Study the drawing (mm; zero at the part's minimum x, y, z) and answer. Round coordinates to 2 decimals unless told otherwise and drop trailing zeros. Order: outer loops, then holes, each group sorted by start corner. A loop starts at its lowest first (then second) coordinate and runs counter-clockwise, first axis right, second up. Notation, with made-up numbers: (-28, 31) - (-10, 31) arc R17 ccw to (-10, 38) - close; hole circle Ø7 at (-15.5, 8). An arc over 180 degrees is marked (long way). Put each result on its own line as item: value.
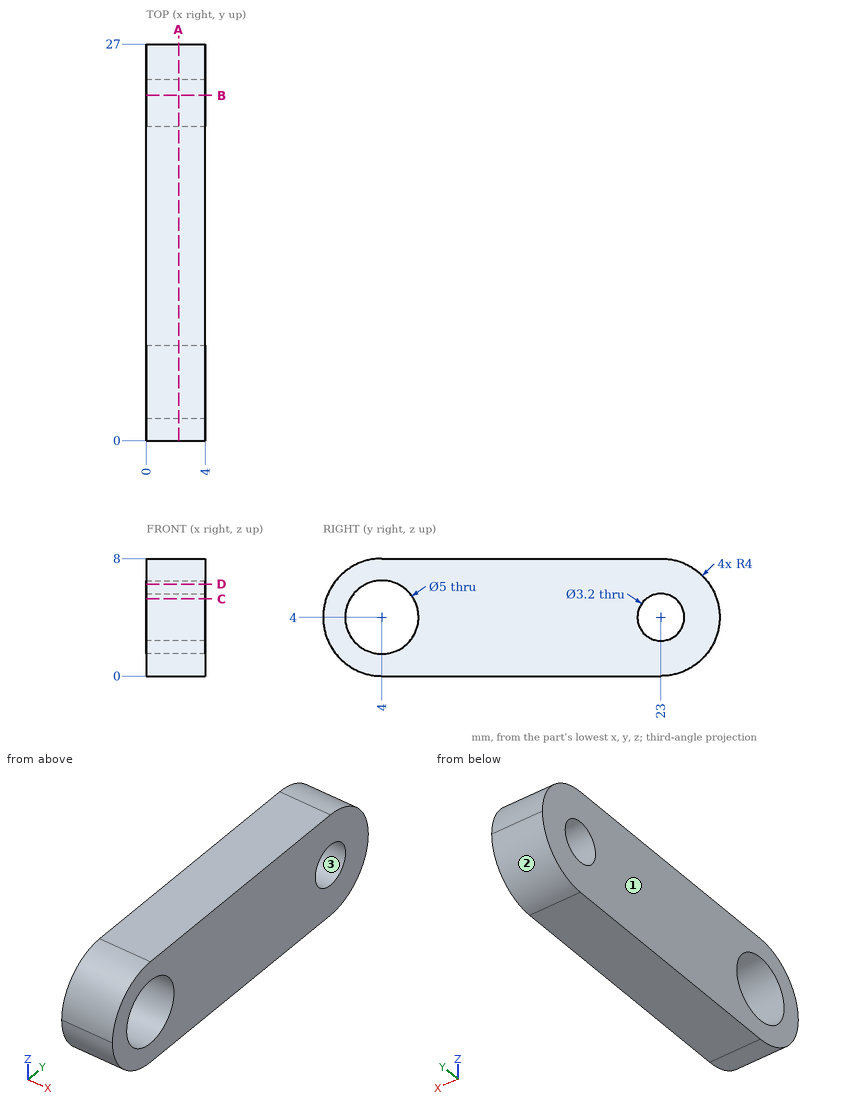
1) A cutting plane is placed at D-D on z = 6.25. Write down the section's boundary in (x, y).
Findings below:
outline: (0, 0.69) - (4, 0.69) - (4, 2.91) - (0, 2.91) - close; (0, 5.09) - (4, 5.09) - (4, 26.31) - (0, 26.31) - close
2) A cutting plane is placed at A-A on x = 2.2. Give the number of separate pieces and of enclosed holes in the cut face, then the cut area to 3 significant figures.
Findings below:
separate pieces: 1
enclosed holes: 2
area: 175 mm2
3) A cutting plane is placed at B-B on y = 23.5. Write down the section's boundary in (x, z), then the cut area to 3 significant figures.
Findings below:
outline: (0, 0.03) - (4, 0.03) - (4, 2.48) - (0, 2.48) - close; (0, 5.52) - (4, 5.52) - (4, 7.97) - (0, 7.97) - close
area: 19.6 mm2
4) Straight lines are drawn through the part: L1, parallel to Y at x = 3.2, z = 4.75 (1 decimal); L2, parallel to Y at x = 0.9, z = 5; L3, parallel to Y at x = 3.25, z = 2. For each, find the intervals that lie inside material, in ascending order. Write a range as from..to.
Findings below:
L1: y = 0.1..1.6, 6.4..21.6, 24.4..26.9
L2: y = 0.13..1.71, 6.29..21.75, 24.25..26.87
L3: y = 0.54..2.5, 5.5..26.46
5) A cutting plane is placed at C-C on z = 5.25. Write down the section's boundary in (x, y) (1 decimal), then the cut area to 3 significant figures.
Findings below:
outline: (0, 0.2) - (4, 0.2) - (4, 1.8) - (0, 1.8) - close; (0, 6.2) - (4, 6.2) - (4, 22) - (0, 22) - close; (0, 24) - (4, 24) - (4, 26.8) - (0, 26.8) - close
area: 81.1 mm2
6) For a pull along Z with two mould halves and no side action, classify the marked faces 1, 2 and 3 as pulls with the +Z half, pulls with the -Z half, needs draft (parallel to the pull), parting line crosses it, or undercut.
Findings below:
face 1: needs draft
face 2: pulls with the -Z half
face 3: undercut
7) Given pin 1 Ø1 at (x, z) = (1.5, 5.5) entering from -Y; pin 2 Ø2 at (x, z) = (1, 7) entering from -Y; pin 3 Ø1.9 at (y, z) = (23, 4) entering from +X, each flat-ended and moving along its own axis, determine where each tip first touches the part or whether it passes through.
Findings below:
pin 1: stops at y = 0.13
pin 2: stops at y = 0.54
pin 3: passes through
